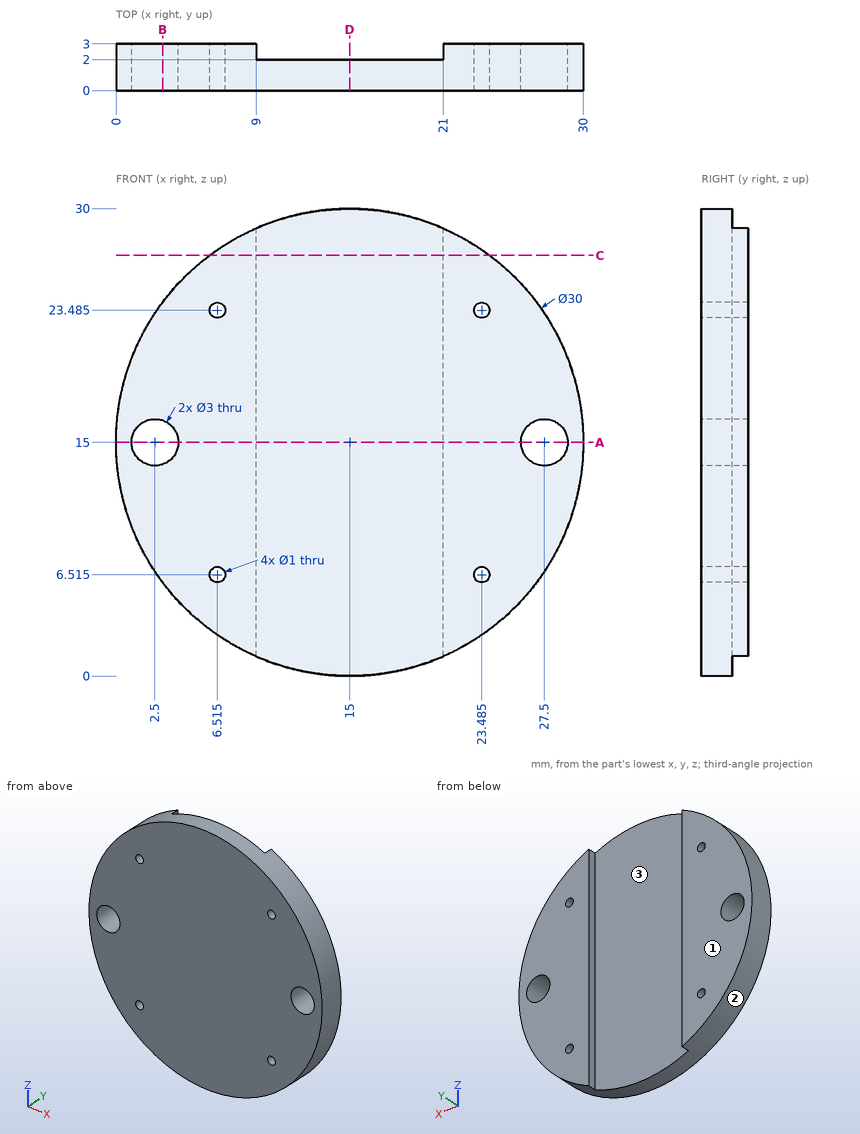
Input: dimensioned drawing with shaded views. Units: mm. Origin: part minimum x, y, z. Round coordinates to 2 decimals unless told otherwise and drop trailing zeros. Order: outer loops, then holes, each group sorted by start corner. A loop starts at its lowest first (then second) coordinate and runs counter-clockwise, first axis right, second up.
1. Cut plane C-C, the plane z = 27. Output: boundary loops of the cut face in (x, y), then the cut area to 3 significant figures.
The answers:
outline: (6, 0) - (24, 0) - (24, 3) - (21, 3) - (21, 2) - (9, 2) - (9, 3) - (6, 3) - close
area: 42.0 mm2
2. Cut plane B-B, the plane x = 3. Output: boundary loops of the cut face in (y, z).
The answers:
outline: (0, 6) - (3, 6) - (3, 13.59) - (0, 13.59) - close; (0, 16.41) - (3, 16.41) - (3, 24) - (0, 24) - close
3. Cut plane A-A, the plane z = 15. Output: boundary loops of the cut face in (x, y), then the cut area to 3 significant figures.
The answers:
outline: (0, 0) - (1, 0) - (1, 3) - (0, 3) - close; (4, 0) - (26, 0) - (26, 3) - (21, 3) - (21, 2) - (9, 2) - (9, 3) - (4, 3) - close; (29, 0) - (30, 0) - (30, 3) - (29, 3) - close
area: 60.0 mm2
4. Pin query (flat end, axial travel): P1, Ø1.5, axis at x = 10, y = 2.5, coming from the -Z side; P2, Ø1.1, axis at y = 2.5, z = 8.5, coming from the +X side; P3, Ø0.5, axis at y = 2.5, z = 13.5, coming from the -X side. Return the tip coordinate at first contact, or that it passes through.
The answers:
P1: stops at z = 0.67
P2: stops at x = 28.77
P3: stops at x = 0.05
5. Mould query, pull axis X, two halves, no side actions, for the marked faces 1, 2 and 3. Classes: released by +X, released by -X, zero draft, split by the parting line, or undercut.
The answers:
face 1: zero draft
face 2: split by the parting line
face 3: undercut
6. Cut plane D-D, the plane x = 15. Output: boundary loops of the cut face in (y, z).
The answers:
outline: (0, 0) - (2, 0) - (2, 30) - (0, 30) - close
7. Material intervals for line 1 (Z direction, x = 23.75, y = 0.2); line 2 (Y direction, x = 16.75, z = 19); line 3 (Z direction, x = 26.5, y = 1.55), sorted ascending.
The answers:
line 1: z = 2.82 to 6.09, 6.94 to 23.06, 23.91 to 27.18
line 2: y = 0 to 2
line 3: z = 5.37 to 13.88, 16.12 to 24.63
